Read the model definition and answer for the solid it produces. Units are mm, in the model's axes. A direction names the side the tool comes from. Give positions to 0.01 mm unless a question says otherwise; leave off trailing zeros. Loops run counter-clockwise (first coordinate to the right, second up) from the corner with the lowest first, then second, coordinate; pieces in that order, holes last. Notation, with made-up numbers: (81.5, -37.5) -> (90.5, -37.5) arc R21 ccw to (90.5, -13.5) -> close; hole circle Ø11 at (88, 21.25). An arc over 180 degrees is marked (long way). One line per item, written item: value. Start each with the question number.
from build123d import *

# Parameters (mm, degrees)
F1_DEPTH    = 245.36945
F2_DEPTH    = 203.2
F3_W        = 163.0290746689
F3_H        = 1246.3291883469
F4_DEPTH    = 635
F5_DEPTH    = 431.8
F6_T1_DEPTH = 2516.4554829813
F7_T1_DEPTH = 2441.5924956103


# Not quite as in the source:
# - a fillet or chamfer that OpenCascade refuses, or shapes differently, is made with other operations: its cross-section is extruded or revolved along the edge and cut away or added


with BuildPart() as f1:
    # F0 (on Front) → F1 (new body)
    with BuildSketch(Plane.XZ):
        with BuildLine():
            Line((-437.8447532654, -40.3878050825), (-437.8447532654, 40.3878050825))
            ThreePointArc((-437.8447532654, 40.3878050825), (-439.703539628, 0), (-437.8447532654, -40.3878050825))
        make_face()
        with BuildLine():
            Line((-437.8447532654, 439.703539628), (-437.8447532654, 40.3878050825))
            Line((-437.8447532654, 40.3878050825), (-437.8447532654, -40.3878050825))
            Line((-437.8447532654, -40.3878050825), (-437.8447532654, -443.3148503304))
            Line((-437.8447532654, -443.3148503304), (0, -443.3148503304))
            Line((0, -443.3148503304), (0, -127))
            ThreePointArc((0, -127), (-127, 0), (0, 127))
            Line((0, 127), (0, 439.703539628))
            Line((0, 439.703539628), (-437.8447532654, 439.703539628))
        make_face()
        with BuildLine():
            Line((440.1807188988, 439.703539628), (0, 439.703539628))
            Line((0, 439.703539628), (0, 127))
            ThreePointArc((0, 127), (89.8025612107, 89.8025612107), (127, 0))
            ThreePointArc((127, 0), (89.8025612107, -89.8025612107), (0, -127))
            Line((0, -127), (0, -443.3148503304))
            Line((0, -443.3148503304), (440.1807188988, -443.3148503304))
            Line((440.1807188988, -443.3148503304), (440.1807188988, 439.703539628))
        make_face()
        with BuildLine():
            Line((0, -127), (0, 127))
            ThreePointArc((0, 127), (-127, 0), (0, -127))
        make_face()
        with BuildLine():
            ThreePointArc((127, 0), (89.8025612107, 89.8025612107), (0, 127))
            Line((0, 127), (0, -127))
            ThreePointArc((0, -127), (89.8025612107, -89.8025612107), (127, 0))
        make_face()
    extrude(amount=F1_DEPTH)

    # F0 (on Front) → F2 (join)
    with BuildSketch(Plane.XZ):
        with BuildLine():
            Line((0, -127), (0, 127))
            ThreePointArc((0, 127), (-127, 0), (0, -127))
        make_face()
        with BuildLine():
            ThreePointArc((127, 0), (89.8025612107, 89.8025612107), (0, 127))
            Line((0, 127), (0, -127))
            ThreePointArc((0, -127), (89.8025612107, -89.8025612107), (127, 0))
        make_face()
    extrude(amount=-F2_DEPTH)

    # F3 (on Front) → F4 (join)
    with BuildSketch(Plane.XZ):
        with Locations((520.3551054001, 6.3239336014)):
            Rectangle(F3_W, F3_H)
    extrude(amount=F4_DEPTH)

    # F3 (on Front) → F5 (join)
    with BuildSketch(Plane.XZ):
        with Locations((520.3551054001, 6.3239336014)):
            Rectangle(F3_W, F3_H)
    extrude(amount=-F5_DEPTH)

    # F6: fillet of radius 457.9913774748 on 1 edges, made by hand

    # F6_s2 → F6_t1 (cut)
    with BuildSketch(Plane.XZ.offset(-1135.5430164906)):
        with BuildLine():
            ThreePointArc((16.3724533309, 439.703539628), (-286.0206379525, 325.6809400755), (-437.8447532654, 40.3878050825))
            Line((-437.8447532654, 40.3878050825), (-437.8447532654, 439.703539628))
            Line((-437.8447532654, 439.703539628), (16.3724533309, 439.703539628))
        make_face()
    extrude(amount=F6_T1_DEPTH, mode=Mode.SUBTRACT)

    # F7: fillet of radius 440.8813389734 on 1 edges, made by hand

    # F7_s2 → F7_t1 (cut)
    with BuildSketch(Plane.XZ.offset(-1098.1115228051)):
        with BuildLine():
            ThreePointArc((-437.8447532654, -40.3878050825), (-296.6295178781, -327.3255664249), (1.3998558567, -443.3148503304))
            Line((1.3998558567, -443.3148503304), (-437.8447532654, -443.3148503304))
            Line((-437.8447532654, -443.3148503304), (-437.8447532654, -40.3878050825))
        make_face()
    extrude(amount=F7_T1_DEPTH, mode=Mode.SUBTRACT)


solid = f1.part
Item 1: Flat-ended cylindrical pins translate along their axes: pin 1 (1 mm diameter, centred on x = 73.5, z = 191, fed in from +Y); pin 2 (4 mm diameter, centred on x = -11.5, y = -211.5, fed in from +Z); pin 3 (10 mm diameter, centred on x = 218, y = -235.5, fed in from -Z). Find the tip coordinate at first contact, or state that the pin passes through.
Item 2: Section B-B, the plane z = 0 is taken. Determine the outline of the cut face in (x, y).
Item 3: Determine the mould class of faces 1 (the flat face through (519, -635, 15)), 2 (the cylindrical face through (-439.703, -120.967, 0.566)), 3 (the cylindrical face through (85.833, 100.178, 93.604)), 4 (the flat face through (601.87, -109, -2)) for opening direction X: pulls with the +X half, pulls with the -X half, needs draft (parallel to the pull), parting line crosses it, or undercut.
Item 4: Section D-D, the plane y = 271.5 is taken. Determine the outline of the cut face in (x, z).
Item 5: For faces 5 (the flat face through (91, 0, -94)), 6 (the flat face through (231, -121, 439.704)), 7 (the flat face through (217, -121, -443.315)), 8 (the flat face through (-7, -245.369, 4)), 9 (the flat face through (-2, 203.2, 2)), determine the directions among +Z, -Z, +X, -X, +Y, -Y from which every point of the face is accessible in a straight line to the end or side of a thin tool.
Item 6: Section A-A, the plane y = 44.5 is taken. Determine the outline of the cut face in (x, z).
Item 7: Section C-C, the plane x = 337.5 is taken. Determine the outline of the cut face in (y, z), plus the area to 3 significant figures.
Item 8: Consider L1, parallel to Y at x = -165.5, z = 246; L2, parallel to X at y = -458, z = 256; L3, parallel to Z at x = 323, y = -151. Determine where each line is inside the solid, lowest interval first. Write a range as [from, to].
Computed values:
1. pin 1: y = 0
1. pin 2: z = 438.97
1. pin 3: z = -443.31
2. outline: (-439.7, -245.37) -> (438.84, -245.37) -> (438.84, -635) -> (601.87, -635) -> (601.87, 431.8) -> (438.84, 431.8) -> (438.84, 0) -> (127, 0) -> (127, 203.2) -> (-127, 203.2) -> (-127, 0) -> (-439.7, 0) -> close
3. face 1: needs draft
3. face 2: pulls with the -X half
3. face 3: undercut
3. face 4: pulls with the +X half
4. outline: (438.84, -616.84) -> (601.87, -616.84) -> (601.87, 629.49) -> (438.84, 629.49) -> close
5. face 5: +Y
5. face 6: +Z, -X, +Y, -Y
5. face 7: -Z, -X, +Y, -Y
5. face 8: +Z, -Z, -X, -Y
5. face 9: +Z, -Z, -X, +Y
6. outline: circle Ø254 at (0, 0); (438.84, -616.84) -> (601.87, -616.84) -> (601.87, 629.49) -> (438.84, 629.49) -> close
7. outline: (-245.37, -443.31) -> (0, -443.31) -> (0, 439.7) -> (-245.37, 439.7) -> close
7. area: 217,000 mm²
8. L1: [-245.37, 0]
8. L2: [438.84, 601.87]
8. L3: [-443.31, 439.7]
